Geometry check sheet. Reference: drawing and pictorial views, mm from the part's lowest x, y, z. A direction names the side the tool comes from. Round coordinates to 2 decimals unless told otherwise and drop trailing zeros. Order: outer loops, then holes, each group sorted by start corner. A loop starts at its lowest first (then second) coordinate and runs counter-clockwise, first axis right, second up.
(1) Sectioned sample at C-C (y = 29). Record the boundary of the cut face in (x, z) (1 decimal).
(2) Release check for a two-part mould opening along Z. For the marked faces 3, 4 and 5 record: +Z half, -Z half, draft (parallel to the pull), parting line (faces both ways), or undercut.
(3) Go/stop test with a flat-tipped pin: pin 1 (9 mm diameter, centred on y = 13.5, z = 6.5, fed in from -X). Record where the tip stops, or that it passes through.
(4) Material ranges on line 1 along Z through (x, y) = (62.5, 17) (1 decimal); line 2 along X through (y, z) = (11, 13.5) (1 decimal), recorded low to high.
(5) Sectioned sample at B-B (z = 5). Record the boundary of the cut face in (x, y) (1 decimal).
(6) Sectioned sample at A-A (x = 81.5). Record the boundary of the cut face in (y, z) (1 decimal).
(7) Set-up check for the marked faces 1 and 2: record each of +Z, -Z, +X, -X, +Y, -Y from which the full face is reachable in a straight line by a thin tool's end or side.
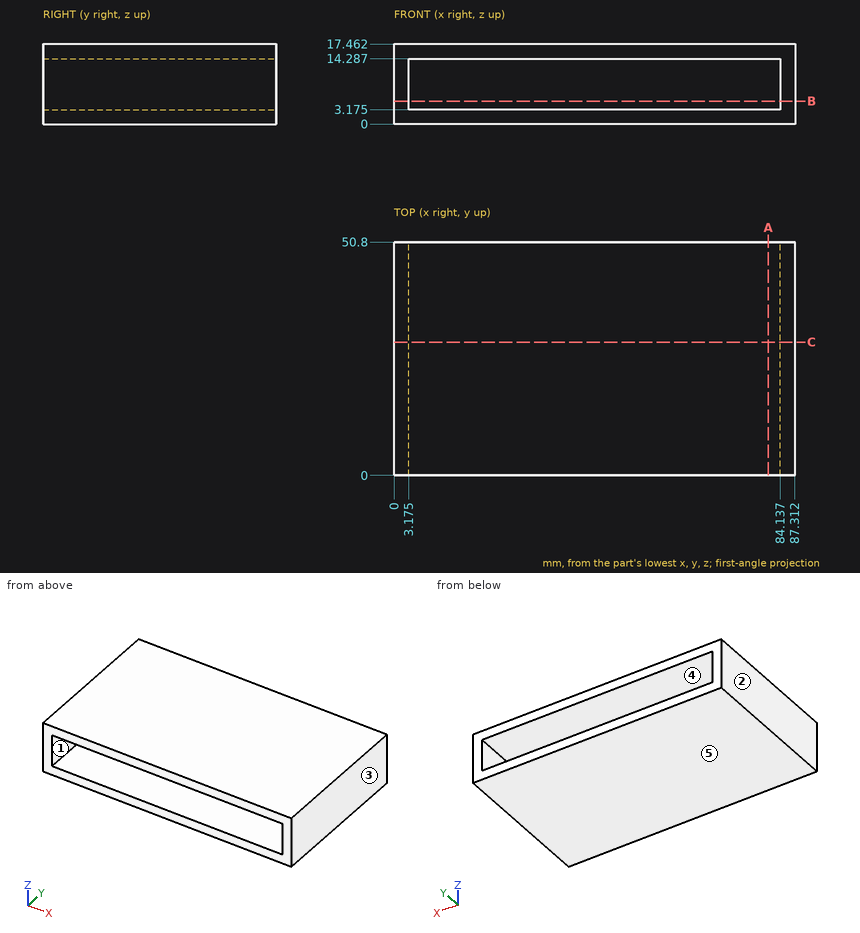
Answer below:
1. outline: (0, 0) - (87.3, 0) - (87.3, 17.5) - (0, 17.5) - close; hole (3.2, 3.2) - (84.1, 3.2) - (84.1, 14.3) - (3.2, 14.3) - close
2. face 3: draft
2. face 4: undercut
2. face 5: -Z half
3. pin 1: stops at x = 0
4. line 1: z = 0 to 3.2, 14.3 to 17.5
4. line 2: x = 0 to 3.2, 84.1 to 87.3
5. outline: (0, 0) - (3.2, 0) - (3.2, 50.8) - (0, 50.8) - close; (84.1, 0) - (87.3, 0) - (87.3, 50.8) - (84.1, 50.8) - close
6. outline: (0, 0) - (50.8, 0) - (50.8, 3.2) - (0, 3.2) - close; (0, 14.3) - (50.8, 14.3) - (50.8, 17.5) - (0, 17.5) - close
7. face 1: +Y, -Y
7. face 2: +Z, -Z, -X, +Y, -Y
